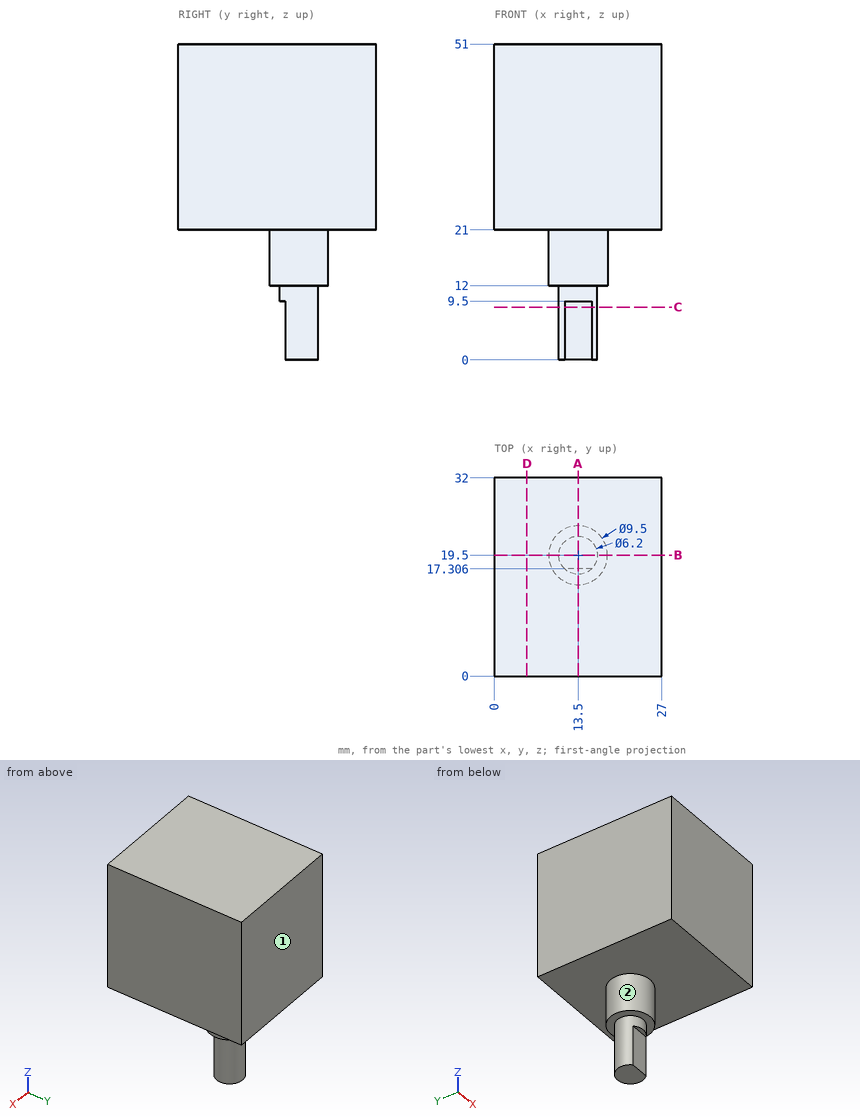
For this review, use the dimensioned drawing (mm, ordinates from the lowest corner) and the shaded views. A direction names the side the tool comes from. Give positions to 0.01 mm unless a question says otherwise; leave off trailing zeros. Order: outer loops, then holes, each group sorted by start corner. A loop starts at its lowest first (then second) coordinate and runs counter-clockwise, first axis right, second up. Notation, with made-up numbers: (-35.5, 78) - (-21.5, 78) arc R25 ccw to (-21.5, 100) - close; hole circle Ø5 at (84.5, -21.75). An arc over 180 degrees is marked (long way). Write item = value, one per line. Start each with the question number.
Q1. Tool access review of the marked faces 1 and 2: name each direction out of +Z, -Z, +X, -X, +Y, -Y from which nothing blocks a thin tool from reaching the whole face with its end or side.
Q2. We need section C-C on z = 8.5. State the section outline as (x, y) points, plus the area to 3 significant figures.
Q3. We need section D-D on x = 5.25. State the section outline as (y, z) points.
Q4. Clearance check with flat-ended pins moving along their axes: pin 1 Ø12 at (x, y) = (19, 12) entering from -Z; pin 2 Ø3 at (x, y) = (15, 17) entering from -Z; pin 3 Ø2 at (x, z) = (13.5, 5.5) entering from -Y; pin 4 Ø1.5 at (y, z) = (18, 7) entering from +X. State where each tip first meets the part, or that it passes through.
Q5. We need section B-B on y = 19.5. State the section outline as (x, z) points, plus the area to 3 significant figures.
Q6. We need section A-A on x = 13.5. State the section outline as (y, z) points.
Q7. To check wall thickness, follow L1, parallel to Z at x = 3, y = 14; L2, parallel to X at y = 19, z = 5.5; L3, parallel to X at y = 16.5, z = 19. State the ranges of each line that lie inside material, in increasing order. Write a range as from..to.
Working result:
q1.face_1 = +Z, -Z, +X, -X, +Y
q1.face_2 = -Z
q2.outline = (11.31, 17.31) - (15.69, 17.31) arc R3.1 ccw (long way) to start
q2.area = 27.5 mm²
q3.outline = (0, 21) - (32, 21) - (32, 51) - (0, 51) - close
q4.pin_1 = 12
q4.pin_2 = 0
q4.pin_3 = 17.31
q4.pin_4 = 16.51
q5.outline = (0, 21) - (8.75, 21) - (8.75, 12) - (10.4, 12) - (10.4, 0) - (16.6, 0) - (16.6, 12) - (18.25, 12) - (18.25, 21) - (27, 21) - (27, 51) - (0, 51) - close
q5.area = 970 mm²
q6.outline = (0, 21) - (14.75, 21) - (14.75, 12) - (16.4, 12) - (16.4, 9.5) - (17.31, 9.5) - (17.31, 0) - (22.6, 0) - (22.6, 12) - (24.25, 12) - (24.25, 21) - (32, 21) - (32, 51) - (0, 51) - close
q7.L1 = 21..51
q7.L2 = 10.44..16.56
q7.L3 = 9.82..17.18
